from build123d import *

# Parameters (mm, degrees)
SKETCH_1_W      = 65.5
SKETCH_1_H      = 65.5
SKETCH_1_R      = 3.6
SKETCH_1_R_2    = 2.55
EXTRUDE_1_DEPTH = 3
FILLET_1_R      = 3


with BuildPart() as part:
    # 草图1 → 凸台-拉伸1 (new body)
    with BuildSketch(Plane(origin=(0, 0, 0), x_dir=(1, 0, 0), z_dir=(0, 1, 0))):
        with Locations((32.75, -32.75)):
            Rectangle(SKETCH_1_W, SKETCH_1_H)
        with Locations(Location((12.9, -12.75, 0), (0, 0, 270))):
            Circle(SKETCH_1_R, mode=Mode.SUBTRACT)
        with Locations(Location((12.9, -32.75, 0), (0, 0, 270))):
            Circle(SKETCH_1_R, mode=Mode.SUBTRACT)
        with Locations(Location((12.9, -52.75, 0), (0, 0, 270))):
            Circle(SKETCH_1_R, mode=Mode.SUBTRACT)
        with Locations(Location((32.75, -32.75, 0), (0, 0, 270))):
            Circle(SKETCH_1_R_2, mode=Mode.SUBTRACT)
        with Locations(Location((22.75, -32.75, 0), (0, 0, 270))):
            Circle(SKETCH_1_R_2, mode=Mode.SUBTRACT)
        with Locations(Location((32.75, -22.75, 0), (0, 0, 270))):
            Circle(SKETCH_1_R_2, mode=Mode.SUBTRACT)
        with Locations(Location((32.75, -42.75, 0), (0, 0, 90))):
            Circle(SKETCH_1_R_2, mode=Mode.SUBTRACT)
        with Locations(Location((42.75, -32.75, 0), (0, 0, 90))):
            Circle(SKETCH_1_R_2, mode=Mode.SUBTRACT)
        with Locations(Location((52.6, -12.75, 0), (0, 0, 270))):
            Circle(SKETCH_1_R_2, mode=Mode.SUBTRACT)
        with Locations(Location((52.6, -22.75, 0), (0, 0, 270))):
            Circle(SKETCH_1_R_2, mode=Mode.SUBTRACT)
        with Locations(Location((52.6, -32.75, 0), (0, 0, 270))):
            Circle(SKETCH_1_R_2, mode=Mode.SUBTRACT)
        with Locations(Location((52.6, -42.75, 0), (0, 0, 270))):
            Circle(SKETCH_1_R_2, mode=Mode.SUBTRACT)
        with Locations(Location((52.6, -52.75, 0), (0, 0, 270))):
            Circle(SKETCH_1_R_2, mode=Mode.SUBTRACT)
        with Locations(Location((12.9, -42.75, 0), (0, 0, 90))):
            Circle(SKETCH_1_R_2, mode=Mode.SUBTRACT)
        with Locations(Location((12.9, -22.75, 0), (0, 0, 90))):
            Circle(SKETCH_1_R_2, mode=Mode.SUBTRACT)
        with BuildLine():
            Line((29.5, -3.55), (36, -3.55))
            ThreePointArc((36, -3.55), (37.5, -5.05), (36, -6.55))
            Line((36, -6.55), (29.5, -6.55))
            ThreePointArc((29.5, -6.55), (28, -5.05), (29.5, -3.55))
        make_face(mode=Mode.SUBTRACT)
        with BuildLine():
            Line((49.35, -3.55), (55.85, -3.55))
            ThreePointArc((55.85, -3.55), (57.35, -5.05), (55.85, -6.55))
            Line((55.85, -6.55), (49.35, -6.55))
            ThreePointArc((49.35, -6.55), (47.85, -5.05), (49.35, -3.55))
        make_face(mode=Mode.SUBTRACT)
        with BuildLine():
            Line((16.15, -3.55), (9.65, -3.55))
            ThreePointArc((9.65, -3.55), (8.15, -5.05), (9.65, -6.55))
            Line((9.65, -6.55), (16.15, -6.55))
            ThreePointArc((16.15, -6.55), (17.65, -5.05), (16.15, -3.55))
        make_face(mode=Mode.SUBTRACT)
        with BuildLine():
            Line((16.15, -61.95), (9.65, -61.95))
            ThreePointArc((9.65, -61.95), (8.15, -60.45), (9.65, -58.95))
            Line((9.65, -58.95), (16.15, -58.95))
            ThreePointArc((16.15, -58.95), (17.65, -60.45), (16.15, -61.95))
        make_face(mode=Mode.SUBTRACT)
        with BuildLine():
            Line((29.5, -61.95), (36, -61.95))
            ThreePointArc((36, -61.95), (37.5, -60.45), (36, -58.95))
            Line((36, -58.95), (29.5, -58.95))
            ThreePointArc((29.5, -58.95), (28, -60.45), (29.5, -61.95))
        make_face(mode=Mode.SUBTRACT)
        with BuildLine():
            Line((49.35, -61.95), (55.85, -61.95))
            ThreePointArc((55.85, -61.95), (57.35, -60.45), (55.85, -58.95))
            Line((55.85, -58.95), (49.35, -58.95))
            ThreePointArc((49.35, -58.95), (47.85, -60.45), (49.35, -61.95))
        make_face(mode=Mode.SUBTRACT)
        with BuildLine():
            Line((22.75, -10.25), (42.75, -10.25))
            ThreePointArc((42.75, -10.25), (45.25, -12.75), (42.75, -15.25))
            Line((42.75, -15.25), (22.75, -15.25))
            ThreePointArc((22.75, -15.25), (20.25, -12.75), (22.75, -10.25))
        make_face(mode=Mode.SUBTRACT)
        with BuildLine():
            Line((22.75, -55.25), (42.75, -55.25))
            ThreePointArc((42.75, -55.25), (45.25, -52.75), (42.75, -50.25))
            Line((42.75, -50.25), (22.75, -50.25))
            ThreePointArc((22.75, -50.25), (20.25, -52.75), (22.75, -55.25))
        make_face(mode=Mode.SUBTRACT)
    extrude(amount=EXTRUDE_1_DEPTH)

    # 圆角1
    fillet_1_edges = [part.edges().sort_by_distance(p)[0] for p in [
        (0, 1.5, 0),
        (65.5, 1.5, 0),
        (65.5, 1.5, 65.5),
        (0, 1.5, 65.5),
    ]]
    fillet(fillet_1_edges, radius=FILLET_1_R)


solid = part.part
Work out the finished part from the listing and answer in its coordinate system (mm). A direction names the side the tool comes from. Coordinates: 2 decimals unless noted, no trailing zeros. Order: outer loops, then holes, each group sorted by start corner. A loop starts at its lowest first (then second) coordinate and runs counter-clockwise, first axis right, second up. Notation, with made-up numbers: (63, 7) - (122, 7) arc R22 ccw to (122, 40) - close; hole circle Ø8 at (22.25, 71.5). An arc over 180 degrees is marked (long way). Put each result on its own line as item: value. Start each with the question number.
1) For a pull along Z with two mould halves and no side action, classify faces 3 (the cylindrical face through (47.85, 1.48, 60.42)), 4 (the flat face through (40, 3, 32)), 5 (the cylindrical face through (0.86, 1.52, 0.9)), 6 (the cylindrical face through (64.6, 1.52, 64.64)) as released by +Z, released by -Z, zero draft, split by the parting line, or undercut.
2) Find section C-C (z = 33). Give the vertices of the cut face in (x, y), plus the area to 3 significant figures.
3) Find section A-A (x = 52.6). State how many separate pieces and enclosed holes the cut face has, plus the area to 3 significant figures.
4) Find section B-B (z = 42.75). Give the vertices of the cut face in (x, y), plus the area to 3 significant figures.
5) Flat-ended cylindrical pins translate along their axes: pin 1 (3 mm diameter, centred on x = 52.5, z = 23, fed in from +Y); pin 2 (8.5 mm diameter, centred on x = 12.9, z = 52.75, fed in from +Y). Find the tip coordinate at first contact, or state that the pin passes through.
6) For faces 1 (the flat face through (32, 1, 0)), 2 (the flat face through (33, 1, 6.55)), determine the directions among +Z, -Z, +X, -X, +Y, -Y from which every point of the face is accessible in a straight line to the end or side of a thin tool.
7) Find the intervals of material crossed by line 1 (X direction, y = 1, z = 42.75); line 2 (X direction, y = 1.95, z = 32.75); line 3 (X direction, y = 2.35, z = 13), in increasing order. Write a range as from..to.
Results list:
1. face 3: undercut
1. face 4: zero draft
1. face 5: released by -Z
1. face 6: released by +Z
2. outline: (0, 0) - (9.31, 0) - (9.31, 3) - (0, 3) - close; (16.49, 0) - (20.21, 0) - (20.21, 3) - (16.49, 3) - close; (25.29, 0) - (30.21, 0) - (30.21, 3) - (25.29, 3) - close; (35.29, 0) - (40.21, 0) - (40.21, 3) - (35.29, 3) - close; (45.29, 0) - (50.06, 0) - (50.06, 3) - (45.29, 3) - close; (55.14, 0) - (65.5, 0) - (65.5, 3) - (55.14, 3) - close
2. area: 114 mm^2
3. separate pieces: 8
3. enclosed holes: 0
3. area: 102 mm^2
4. outline: (0, 0) - (10.35, 0) - (10.35, 3) - (0, 3) - close; (15.45, 0) - (30.2, 0) - (30.2, 3) - (15.45, 3) - close; (35.3, 0) - (50.05, 0) - (50.05, 3) - (35.3, 3) - close; (55.15, 0) - (65.5, 0) - (65.5, 3) - (55.15, 3) - close
4. area: 151 mm^2
5. pin 1: passes through
5. pin 2: stops at y = 3
6. face 1: -Z, +X, -X, +Y, -Y
6. face 2: +Y, -Y
7. line 1: x = 0..10.35, 15.45..30.2, 35.3..50.05, 55.15..65.5
7. line 2: x = 0..9.3, 16.5..20.2, 25.3..30.2, 35.3..40.2, 45.3..50.05, 55.15..65.5
7. line 3: x = 0..9.31, 16.49..20.26, 45.24..50.06, 55.14..65.5
